```python
from build123d import *

# Parameters (mm, degrees)
SKETCH1_R               = 25
BOSS_EXTRUDE5_DEPTH     = 20
CUT_EXTRUDE2_DEPTH      = 1
CUT_EXTRUDE2_DEPTH_BACK = 5
SKETCH5_R               = 20
SKETCH9_R               = 15
CUT_EXTRUDE3_DEPTH      = 29


with BuildPart() as part:
    # Sketch1 → Boss-Extrude5 (new body)
    with BuildSketch(Plane(origin=(0, 0, 0), x_dir=(1, 0, 0), z_dir=(0, 1, 0))):
        with Locations(Location((0, 0, 0), (0, 0, 270))):
            Circle(SKETCH1_R)
    extrude(amount=BOSS_EXTRUDE5_DEPTH)

    # Sketch5 → Cut-Extrude2 (cut, two sides: drawn at the far end of the back side and taken through both)
    with BuildSketch(Plane(origin=(0, 20, 0), x_dir=(1, 0, 0), z_dir=(0, 1, 0)).offset(-CUT_EXTRUDE2_DEPTH_BACK)):
        with Locations(Location((0.202413874, 0.104402365, 0), (0, 0, 270))):
            Circle(SKETCH5_R)
    extrude(amount=CUT_EXTRUDE2_DEPTH + CUT_EXTRUDE2_DEPTH_BACK, mode=Mode.SUBTRACT)

    # Sketch9 → Cut-Extrude3 (cut)
    with BuildSketch(Plane(origin=(0, 15, 0), x_dir=(1, 0, 0), z_dir=(0, 1, 0))):
        with Locations(Location((0, 0, 0), (0, 0, 270))):
            Circle(SKETCH9_R)
    extrude(amount=-CUT_EXTRUDE3_DEPTH, mode=Mode.SUBTRACT)


solid = part.part
```
Geometry: final body of the model. Coordinates: model frame, mm. A direction names the side the tool comes from. Coordinates: 2 decimals unless noted, no trailing zeros. Loops run counter-clockwise (first coordinate to the right, second up) from the corner with the lowest first, then second, coordinate; pieces in that order, holes last. Notation, with made-up numbers: M 1.25,4.5 L 30.25,4.5 A32 ccw 30.25,33.5 Z; hole C 72.5,-8 d4. An arc over 180 degrees is marked long. Put each result on its own line as item: value.
(1) Draft query along Z for faces 1 (the face through (0.66, 7.605, -14.985)), 2 (the face through (-19.32, 17.46, -4.44)), 3 (the face through (7.509, 9.86, 23.846)), 4 (the face through (-20, 20, -2)). Return one class per face: pulls with the +Z half, pulls with the -Z half, needs draft (parallel to the pull), parting line crosses it, or undercut.
Answer sheet:
face 1: undercut
face 2: undercut
face 3: parting line crosses it
face 4: needs draft
(2) First-contact query: pin 1 (5 mm diameter, centred on x = -14.5, z = -1.5, fed in from +Y); pin 2 (8 mm diameter, centred on y = 11.5, z = -8, fed in from +X); pin 3 (8 mm diameter, centred on y = 17.5, z = 1.5, fed in from +X); pin 4 (8 mm diameter, centred on x = -3, y = 16.5, fed in from +Z). Flat tips, straight axial feed; report the tip coordinate or a pass-through.
Answer sheet:
pin 1: stops at y = 15
pin 2: stops at x = 24.68
pin 3: stops at x = 25
pin 4: stops at z = 25
(3) Cut plane C-C on y = 5.25. Return the cut outline in (x, z).
Answer sheet:
outline: C 0,0 d50; hole C 0,0 d30
(4) Cut plane A-A on x = 10.5. Return the cut outline in (y, z).
Answer sheet:
outline: M 0,-22.69 L 20,-22.69 L 20,-17.25 L 15,-17.25 L 15,-10.71 L 0,-10.71 Z; M 0,10.71 L 15,10.71 L 15,17.04 L 20,17.04 L 20,22.69 L 0,22.69 Z
(5) Cut plane B-B on z = 0. Return the cut outline in (x, y), then the cut area to 3 significant figures.
Answer sheet:
outline: M -25,0 L -15,0 L -15,15 L -19.8,15 L -19.8,20 L -25,20 Z; M 15,0 L 25,0 L 25,20 L 20.2,20 L 20.2,15 L 15,15 Z
area: 350 mm^2
(6) Cut plane D-D on y = 16.25. Return the cut outline in (x, z), then the cut area to 3 significant figures.
Answer sheet:
outline: C 0,0 d50; hole C 0.2,-0.1 d40
area: 707 mm^2
(7) Access query for faces 5 (the face through (-13, 15, -8)), 6 (the face through (-11, 0, 11)). Directions: +Z, -Z, +X, -X, +Y, -Y. A direction counts if a zero-diameter tool reaches every point of the face in a straight line with its end or side. Return the directions, or none.
Answer sheet:
face 5: +Y
face 6: +Z, -Z, +X, -X, -Y
(8) Material intervals for probe 1 along X at (y, z) = (6.75, 0); probe 2 along Y at (x, z) = (-19, 1); probe 3 along Z at (x, y) = (-6, 4.5), sorted ascending.
Answer sheet:
probe 1: x = -25 to -15, 15 to 25
probe 2: y = 0 to 15
probe 3: z = -24.27 to -13.75, 13.75 to 24.27
